Check sheet for the modelled part. Datum: model origin and axes. Units: mm. Face numbers are marked on the shaded views. A direction names the side the tool comes from. Round coordinates to 2 decimals unless told otherwise and drop trailing zeros. Write each loop counter-clockwise with the first axis right and the second up, starting at its lowest first coordinate (ties: lowest second). Pieces come first, ordered by that corner, then holes.
Item 1: Section check A-A, the plane z = 0.5. Record the cut outline in (x, y).
Item 2: Section check B-B, the plane x = 9.25. Record the cut outline in (y, z).
Item 3: Set-up check for the marked faces 1 and 2: record each of +Z, -Z, +X, -X, +Y, -Y from which the full face is reachable in a straight line by a thin tool's end or side.
Item 4: Release check for a two-part mould opening along Y. For the marked faces 3, 4 and 5 record: pulls with the +Y half, pulls with the -Y half, needs draft (parallel to the pull), parting line crosses it, or undercut.
Item 5: Material ranges on line 1 along Z through (x, y) = (-9.25, -16); line 2 along Y through (x, z) = (-6.5, -2.5); line 3 along X through (y, z) = (-18, 0), recorded low to high.
Item 6: Depth check by flat-ended pin: pin 1 (5 mm diameter, centred on x = 4.5, z = -9, fed in from -Y). Enter the tip coordinate at first touch or a pass-through.
Item 7: Section check D-D, the plane x = 0. Record the cut outline in (y, z), plus the area to 4 significant figures.
Item 8: Section check C-C, the plane z = 21.25. Record the cut outline in (x, y), plus the area to 4 significant figures.
from build123d import *

# Parameters (mm, degrees)
F0_W     = 22.5
F0_H     = 65
F0_R     = 1.5
F1_DEPTH = 25
F2_R     = 3.5
F3_DEPTH = 10


with BuildPart() as f1:
    # F0 (on Front) → F1 (new body)
    with BuildSketch(Plane.XZ):
        Rectangle(F0_W, F0_H)
        with Locations((-9.25, 0.5)):
            Circle(F0_R, mode=Mode.SUBTRACT)
        with Locations((9.25, 0.5)):
            Circle(F0_R, mode=Mode.SUBTRACT)
    extrude(amount=F1_DEPTH)

    # F2 (on face) → F3 (join)
    with BuildSketch(Plane.XZ.offset(25)):
        with Locations((0, 21.25)):
            Circle(F2_R)
    extrude(amount=F3_DEPTH)


solid = f1.part
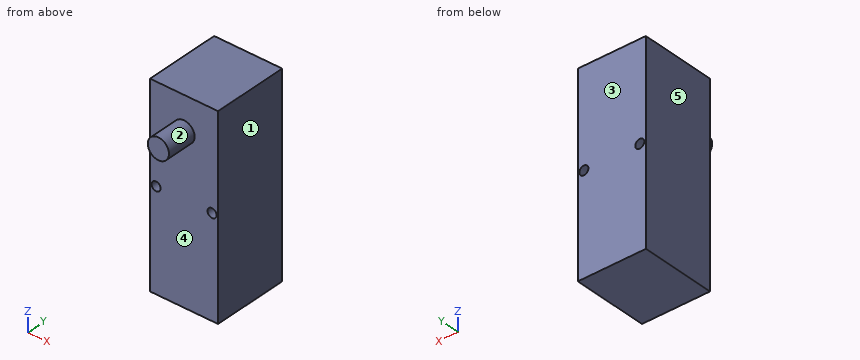
Values found:
1. outline: (-11.25, -25) - (-10.75, -25) - (-10.75, 0) - (-11.25, 0) - close; (-7.75, -25) - (7.75, -25) - (7.75, 0) - (-7.75, 0) - close; (10.75, -25) - (11.25, -25) - (11.25, 0) - (10.75, 0) - close
2. outline: (-25, -32.5) - (0, -32.5) - (0, -1) - (-25, -1) - close; (-25, 2) - (0, 2) - (0, 32.5) - (-25, 32.5) - close
3. face 1: +Z, -Z, +X, +Y, -Y
3. face 2: -Y
4. face 3: pulls with the +Y half
4. face 4: pulls with the -Y half
4. face 5: needs draft
5. line 1: z = -32.5 to -1, 2 to 32.5
5. line 2: y = -25 to 0
5. line 3: x = -11.25 to -10.66, -7.84 to 7.84, 10.66 to 11.25
6. pin 1: stops at y = -25
7. outline: (-35, 17.75) - (-25, 17.75) - (-25, -32.5) - (0, -32.5) - (0, 32.5) - (-25, 32.5) - (-25, 24.75) - (-35, 24.75) - close
7. area: 1,695 mm2
8. outline: (-11.25, -25) - (-3.5, -25) - (-3.5, -35) - (3.5, -35) - (3.5, -25) - (11.25, -25) - (11.25, 0) - (-11.25, 0) - close
8. area: 632.5 mm2
